from build123d import *

# Parameters (mm, degrees)
SKETCH1_R               = 23.25
BOSS_EXTRUDE1_DEPTH     = 5
CUT_EXTRUDE1_DEPTH      = 34.258457571
CIRPATTERN1_COUNT       = 29
CUT_EXTRUDE2_DEPTH      = 35.357810434
CUT_EXTRUDE2_DEPTH_BACK = 35.357810434
SKETCH3_R               = 4.25
SKETCH4_R               = 2.1
CUT_EXTRUDE3_DEPTH      = 35.357810434
CIRPATTERN2_COUNT       = 4


with BuildPart() as part:
    # Sketch1 → Boss-Extrude1 (new, symmetric)
    with BuildSketch(Plane(origin=(0, 0, 0), x_dir=(1, 0, 0), z_dir=(0, 1, 0))):
        with Locations(Location((0, 0, 0), (0, 0, 270))):
            Circle(SKETCH1_R)
    extrude(amount=BOSS_EXTRUDE1_DEPTH, both=True)

    # Sketch2 → Cut-Extrude1 (cut, symmetric)
    with BuildSketch(Plane(origin=(0, 0, 0), x_dir=(1, 0, 0), z_dir=(0, 1, 0))):
        with BuildLine():
            ThreePointArc((0.696879992, 19.861778225), (0, 19.874), (-0.696879992, 19.861778225))
            ThreePointArc((-0.696879992, 19.861778225), (-1.219525976, 21.594414991), (-2.089327454, 23.181435589))
            ThreePointArc((-2.089327454, 23.181435589), (0, 23.2754), (2.089327454, 23.181435589))
            ThreePointArc((2.089327454, 23.181435589), (1.219525976, 21.594414991), (0.696879992, 19.861778225))
        make_face()
    cut_extrude1 = extrude(amount=CUT_EXTRUDE1_DEPTH, both=True, mode=Mode.SUBTRACT)

    # CirPattern1: Cut-Extrude1 ×29 about axis
    cirpattern1_axis = Axis((0, 0, 0), (0, 1, 0))
    for i in range(1, CIRPATTERN1_COUNT):
        add(cut_extrude1.rotate(cirpattern1_axis, i * 360 / CIRPATTERN1_COUNT), mode=Mode.SUBTRACT)

    # Sketch3 → Cut-Extrude2 (cut, two sides: drawn at the far end of the back side and taken through both)
    with BuildSketch(Plane(origin=(0, 5, 0), x_dir=(1, 0, 0), z_dir=(0, 1, 0)).offset(-CUT_EXTRUDE2_DEPTH_BACK)):
        with Locations(Location((0, 0, 0), (0, 0, 270))):
            Circle(SKETCH3_R)
    extrude(amount=CUT_EXTRUDE2_DEPTH + CUT_EXTRUDE2_DEPTH_BACK, mode=Mode.SUBTRACT)

    # Sketch4 → Cut-Extrude3 (cut, symmetric)
    with BuildSketch(Plane(origin=(0, 5, 0), x_dir=(1, 0, 0), z_dir=(0, 1, 0))):
        with Locations(Location((0, -12, 0), (0, 0, 270))):
            Circle(SKETCH4_R)
    cut_extrude3 = extrude(amount=CUT_EXTRUDE3_DEPTH, both=True, mode=Mode.SUBTRACT)

    # CirPattern2: Cut-Extrude3 ×4 about axis
    cirpattern2_axis = Axis((0, 0, 0), (0, 1, 0))
    for i in range(1, CIRPATTERN2_COUNT):
        add(cut_extrude3.rotate(cirpattern2_axis, i * 360 / CIRPATTERN2_COUNT), mode=Mode.SUBTRACT)


solid = part.part
The listing builds one solid part. Answer for the finished solid, in the listing's coordinates (mm). A direction names the side the tool comes from. Give positions to 0.01 mm unless a question says otherwise; leave off trailing zeros. One line per question, with ' | ' between items. Start each with the question number.
1. Section A-A, the plane y = -1.5 is taken. Count the separate pieces of the cut face and the enclosed holes in it, then the cut area to 3 significant figures.
2. For faces 4 (the face through (18.48, 0.07, -11.16)), 5 (the face through (10.09, 0.07, 19.14)), 6 (the face through (10.18, 0.07, -19.09)), 7 (the face through (-18.514, 0.07, -11.201)), determine the directions among +Z, -Z, +X, -X, +Y, -Y from which every point of the face is accessible in a straight line to the end or side of a thin tool.
3. Straight lines are drawn through the part: line 1 (X direction, y = -1.75, z = 12); line 2 (X direction, y = -3.5, z = 1.5); line 3 (X direction, y = 3.75, z = 13). For each, find the intervals that lie inside material, in ascending order.
4. Given P1, Ø5, axis at x = -16.5, y = 1.5, coming from the -Z side; P2, Ø4, axis at x = 7.5, y = 1.5, coming from the -Z side; P3, Ø3, axis at y = -4, z = -5, coming from the +X side; P4, Ø3.5, axis at x = 0, z = -12, coming from the +Y side, each flat-ended and moving along its own axis, determine where each tip first touches the part or whether it passes through.
5. Determine the mould class of faces 1 (the face through (-10.08, 0.07, 19.09)), 2 (the face through (0, -5, 5)), 3 (the face through (8.02, 0.07, 20.04)) for opening direction Z: +Z half, -Z half, draft (parallel to the pull), parting line (faces both ways), or undercut.
Result:
1) separate pieces: 1 | enclosed holes: 5 | area: 1,340 mm2
2) face 4: +X, +Y, -Y | face 5: +Y, -Y | face 6: -Z, +Y, -Y | face 7: -X, +Y, -Y
3) line 1: x = -16.31 to -2.1, 2.1 to 16.31 | line 2: x = -23.2 to -13.47, -10.53 to -3.98, 3.98 to 10.53, 13.47 to 23.2 | line 3: x = -17.1 to -1.85, 1.85 to 17.1
4) P1: stops at z = -17.18 | P2: stops at z = -22.17 | P3: stops at x = 22.99 | P4: passes through
5) face 1: undercut | face 2: draft | face 3: +Z half
